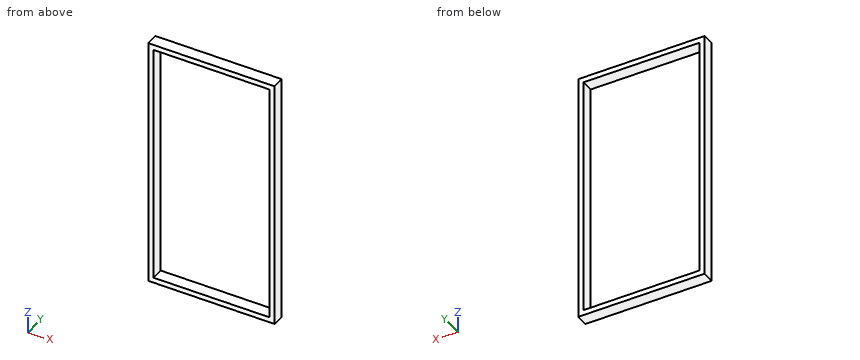
Autodesk Fusion 360 part; units mm, degrees
sketch "Sketch1" plane through (0, 0, 0) normal (0, 0, 1) x (1, 0, 0)
  line L0 (-121.92, 12.192) -> (792.48, 12.192)
  line L1 (792.48, 12.192) -> (792.48, -76.708)
  line L2 (792.48, -76.708) -> (-121.92, -76.708)
  line L3 (-121.92, -76.708) -> (-121.92, 12.192)
  dimension "d1" = 914.4
  dimension "d6" = 88.9
extrude "Extrude1" add sketch "Sketch1" along normal blind 38.1
sketch "Sketch2" plane through (0, 0, 38.1) normal (0, 0, 1) x (-1, 0, 0)
  line L0 (121.92, 76.708) -> (-792.48, 76.708)
  line L1 (-792.48, 76.708) -> (-792.48, -12.192)
  line L2 (-792.48, -12.192) -> (121.92, -12.192)
  line L3 (121.92, -12.192) -> (121.92, 76.708)
  line L4 (121.92, -12.192) -> (83.82, -12.192)
  line L5 (83.82, -12.192) -> (83.82, 76.708)
  line L6 (83.82, 76.708) -> (121.92, 76.708)
  line L7 (121.92, 76.708) -> (121.92, -12.192)
  line L8 (-792.48, -12.192) -> (-754.38, -12.192)
  line L9 (-754.38, -12.192) -> (-754.38, 76.708)
  line L10 (-754.38, 76.708) -> (-792.48, 76.708)
  line L11 (-792.48, 76.708) -> (-792.48, -12.192)
  dimension "d9" = 38.1
  dimension "d10" = 38.1
extrude "Extrude2" add sketch "Sketch2" along normal blind 1752.6 contours L0 L2 L3 L4 L5 L6 L7 | L0 L1 L2 L8 L9 L10 L11
sketch "Sketch3" plane through (0, 0, 1790.7) normal (0, 0, 1) x (-1, 0, 0)
  line L0 (121.92, 76.708) -> (83.82, 76.708)
  line L1 (83.82, 76.708) -> (83.82, -12.192)
  line L2 (83.82, -12.192) -> (121.92, -12.192)
  line L3 (121.92, -12.192) -> (121.92, 76.708)
  line L4 (121.92, 76.708) -> (-792.48, 76.708)
  line L5 (-792.48, 76.708) -> (-792.48, -12.192)
  line L6 (-792.48, -12.192) -> (121.92, -12.192)
  line L7 (121.92, -12.192) -> (121.92, 76.708)
  dimension "d13" = 88.9
  dimension "d14" = 914.4
extrude "Extrude3" add sketch "Sketch3" along normal blind 38.1
sketch "Sketch4" plane through (0, -76.708, 0) normal (0, -1, 0) x (1, 0, 0)
  line L0 (754.38, 1790.7) -> (754.38, 38.1)
  line L1 (754.38, 38.1) -> (-83.82, 38.1)
  line L2 (-83.82, 38.1) -> (-83.82, 1790.7)
  line L3 (-83.82, 1790.7) -> (754.38, 1790.7)
  line L4 (792.48, 0) -> (792.48, 1828.8)
  line L5 (792.48, 1828.8) -> (-121.92, 1828.8)
  line L6 (-121.92, 1828.8) -> (-121.92, 0)
  line L7 (-121.92, 0) -> (792.48, 0)
  line L8 (-121.92, 1828.8) -> (792.48, 1828.8)
  line L9 (792.48, 1828.8) -> (792.48, 0)
  line L10 (792.48, 0) -> (-121.92, 0)
  line L11 (-121.92, 0) -> (-121.92, 1828.8)
  dimension "d17" = 914.4
  dimension "d18" = 1828.8
equation "d1 = BottomLength / 2"
equation "BottomLength = 6 ft"
equation "TopLength = 6 ft"
equation "RightLength = 6 ft"
equation "LeftLength = 6 ft"
equation "d11 = RightLength - ( ( ( 2 * 1.5 ) / 12 ) * 1 ft )"
equation "d14 = TopLength / 2"
Verification items for the finished model (mm, model axes). Give positions to 0.01 mm unless a question says otherwise; leave off trailing zeros. Order: outer loops, then holes, each group sorted by start corner. A loop starts at its lowest first (then second) coordinate and runs counter-clockwise, first axis right, second up. Notation, with made-up numbers: (14, -1.75) - (42, -1.75) arc R30 cw to (42, 37.25) - close; hole circle Ø10 at (-33.5, -26.5). An arc over 180 degrees is marked (long way). Answer as CSV lines item,"result". Start each with the question number.
Item 1: Material ranges on L1, parallel to Z at x = 52, y = -7.5; L2, parallel to X at y = -23, z = 372, recorded low to high.
Item 2: Section check C-C, the plane z = 561.5. Record the boundary of the cut face in (x, y), plus the area to 3 significant figures.
Item 3: Section check A-A, the plane y = -28.5. Record the boundary of the cut face in (x, z).
Item 4: Section check B-B, the plane x = 671. Record the boundary of the cut face in (y, z).
Filled in:
1,L1,"0 to 38.1, 1790.7 to 1828.8"
1,L2,"-121.92 to -83.82, 754.38 to 792.48"
2,outline,"(-121.92, -76.71) - (-83.82, -76.71) - (-83.82, 12.19) - (-121.92, 12.19) - close; (754.38, -76.71) - (792.48, -76.71) - (792.48, 12.19) - (754.38, 12.19) - close"
2,area,"6,770 mm^2"
3,outline,"(-121.92, 0) - (792.48, 0) - (792.48, 1828.8) - (-121.92, 1828.8) - close; hole (-83.82, 38.1) - (754.38, 38.1) - (754.38, 1790.7) - (-83.82, 1790.7) - close"
4,outline,"(-76.71, 0) - (12.19, 0) - (12.19, 38.1) - (-76.71, 38.1) - close; (-76.71, 1790.7) - (12.19, 1790.7) - (12.19, 1828.8) - (-76.71, 1828.8) - close"
